Geometry: final body of the model. Coordinates: model frame, mm. A direction names the side the tool comes from. Round coordinates to 2 decimals unless told otherwise and drop trailing zeros. Write each loop counter-clockwise with the first axis right and the second up, starting at its lowest first coordinate (ties: lowest second). Pieces come first, ordered by that corner, then holes. Notation, with made-up numbers: (-24.75, 23) - (11.25, 23) arc R18 ccw to (11.25, 50) - close; hole circle Ø1 at (-38, 26). An arc over 180 degrees is marked (long way). Use a Markdown table: item, result. Add a question column.
Autodesk Inventor part; units mm, degrees
ref_plane "YZ Plane" through (0, 0, 0) normal (1, 0, 0) x (0, 1, 0)
ref_plane "XZ Plane" through (0, 0, 0) normal (0, 1, 0) x (-1, 0, 0)
ref_plane "XY Plane" through (0, 0, 0) normal (0, 0, 1) x (1, 0, 0)
sketch "Esquisse1" plane through (0, 0, 0) normal (0, 1, 0) x (-1, 0, 0)
  line L0 (22.5, 38.9711) -> (30, 51.9615)
  line L1 (0, 0) -> (55, 0) construction
  line L2 (-22.5, 38.9711) -> (-30, 51.9615)
  line L3 (0, 0) -> (55, 0) construction
  line L4 (0, -65) -> (10, -65)
  line L5 (10, -65) -> (10, -43.8748)
  line L6 (0, -65) -> (-10, -65)
  line L7 (-10, -65) -> (-10, -43.8748)
  line L8 (27.4019, 53.4615) -> (18.3483, 37.7802)
  arc A0 (-18.3483, 37.7802) -> (18.3483, 37.7802) centre (0, 0) ccw
  line L9 (-18.3483, 37.7802) -> (-27.4019, 53.4615)
  line L10 (27.4019, 53.4615) -> (30, 51.9615)
  line L11 (-30, 51.9615) -> (-27.4019, 53.4615)
  arc A1 (-22.5, 38.9711) -> (-10, -43.8748) centre (0, 0) ccw
  arc A2 (10, -43.8748) -> (22.5, 38.9711) centre (0, 0) ccw
  dimension "d1" = 60
  dimension "d2" = 60
  dimension "d3" = 60
  dimension "d4" = 120
extrude "Extrusion1" add sketch "Esquisse1" along normal blind 25
sketch "Esquisse2" plane through (10, 0, -43.8748) normal (1, 0, 0) x (0, 0, -1)
  line L0 (0, 25) -> (21.1252, 25)
  line L1 (21.1252, 25) -> (2.2112, 102.732)
  line L2 (2.2112, 102.732) -> (2.2112, 112.732)
  line L3 (0, 112.732) -> (0, 102.4668)
  line L4 (0, 102.4668) -> (18.8494, 25)
  line L5 (0, 112.732) -> (2.2112, 112.732)
  point P0 (-43.8748, 0)
  dimension "d11" = 80
  dimension "d12" = 10
extrude "Extrusion2" add sketch "Esquisse2" against normal blind 20
fillet "Congé1" radius 2 1 edges at (0, 25, -62.7243)
fillet "Congé2" radius 2 2 edges at (10, 12.5, -43.8748) (-10, 12.5, -43.8748)
fillet "Congé3" radius 2 4 edges at (18.3483, 12.5, 37.7802) (-18.3483, 12.5, 37.7802) (22.5, 12.5, 38.9711) (-22.5, 12.5, 38.9711)
properties part number "omikuji"
1) Section C-C, the plane x = -31.5. Return the cut outline in (y, z).
2) Draft query along X for faces 1 (the flat face through (26.69, 12.32, 46.23)), 2 (the flat face through (-10, 25, -41)), 3 (the cylindrical face through (-1.55, 12.32, -41.97)), 4 (the flat face through (23.34, 12.32, 46.43)). Return one class per face: released by +X, released by -X, zero draft, split by the parting line, or undercut.
3) Section D-D, the plane x = 0. Return the cut outline in (y, z), then the cut area to 3 significant figures.
4) Pin query (flat end, axial travel): P1, Ø12, axis at x = 21.5, y = 83.5, coming from the +Z side; P2, Ø17, axis at y = 61, z = -53.5, coming from the +X side; P3, Ø12, axis at x = 4.5, y = 82.5, coming from the -Z side; P4, Ø3, axis at x = -3.5, y = 108.5, coming from the -Z side. Return the tip coordinate at first contact, or that it passes through.
5) Section A-A, the plane z = 0. Return the cut outline in (x, y), then the cut area to 3 significant figures.
6) Set-up query: faces 5 (the flat face through (-26.69, 12.32, 46.23)), 6 (the flat face through (0, 108, -46.086)), 7 (the flat face through (0, 108, -43.875)). Return all of +Z, -Z, +X, -X, +Y, -Y with unobstructed straight access to the full face (end or side cutting, diameter ignored); none if empty.
7) Section B-B, the plane y = 18. Return the cut outline in (x, z), then the cut area to 3 significant figures.
8) Material intervals for L1, parallel to X at y = 20, z = 0; L2, parallel to Z at x = 0, y = 13.25; L3, parallel to X at y = 16.5, z = 25.5, sorted ascending. Write a range as from..to.
Output values:
| question | item | result |
|---|---|---|
| 1 | outline | (0, -32.14) - (25, -32.14) - (25, -27.78) - (0, -27.78) - close; (0, 27.78) - (25, 27.78) - (25, 32.14) - (0, 32.14) - close |
| 2 | face 1 | released by +X |
| 2 | face 2 | zero draft |
| 2 | face 3 | undercut |
| 2 | face 4 | undercut |
| 3 | outline | (0, -65) - (25, -65) - (102.73, -46.09) - (112.73, -46.09) - (112.73, -43.87) - (102.47, -43.87) - (27.47, -62.12) arc R2 cw to (25, -60.18) - (25, -42) - (0, -42) - close |
| 3 | area | 775 mm^2 |
| 4 | P1 | passes through |
| 4 | P2 | stops at x = 10 |
| 4 | P3 | stops at z = -52.47 |
| 4 | P4 | stops at z = -46.09 |
| 5 | outline | (-45, 0) - (-42, 0) - (-42, 25) - (-45, 25) - close; (42, 0) - (45, 0) - (45, 25) - (42, 25) - close |
| 5 | area | 150 mm^2 |
| 6 | face 5 | -X, +Y, -Y |
| 6 | face 6 | -Z, +X, -X, +Y |
| 6 | face 7 | +Z, +X, -X, +Y |
| 7 | outline | (-30, 51.96) - (-23.48, 40.67) arc R2 cw to (-24.14, 37.98) arc R45 ccw to (-11.49, -43.51) arc R2 cw to (-10, -45.44) - (-10, -65) - (10, -65) - (10, -45.44) arc R2 cw to (11.49, -43.51) arc R45 ccw to (24.14, 37.98) arc R2 cw to (23.48, 40.67) - (30, 51.96) - (27.4, 53.46) - (19.4, 39.6) arc R2 ccw to (20.17, 36.84) arc R42 cw (long way) to (-20.17, 36.84) arc R2 ccw to (-19.4, 39.6) - (-27.4, 53.46) - close |
| 7 | area | 1,200 mm^2 |
| 8 | L1 | x = -45..-42, 42..45 |
| 8 | L2 | z = -65..-42 |
| 8 | L3 | x = -37.08..-33.37, 33.37..37.08 |
